from build123d import *

# Parameters (mm, degrees)
F0_W     = 119
F0_H     = 150.5
F1_DEPTH = 22
F2_W     = 109
F2_H     = 140.5
F3_DEPTH = 15
F5_DEPTH = 25
F7_DEPTH = 4


with BuildPart() as f1:
    # F0 (on Front) → F1 (new body)
    with BuildSketch(Plane.XZ):
        Rectangle(F0_W, F0_H)
    extrude(amount=F1_DEPTH)

    # F2 (on face) → F3 (cut)
    with BuildSketch(Plane.XZ.offset(22)):
        Rectangle(F2_W, F2_H)
    extrude(amount=-F3_DEPTH, mode=Mode.SUBTRACT)

    # F4 (on face) → F5 (cut)
    with BuildSketch(Plane.YZ.offset(59.5)):
        Polygon((-22, 65.25), (-22, 0), (-22, -65.25), (-12, -65.25), (-12, 0), (-12, 65.25), align=None)
    extrude(amount=-F5_DEPTH, mode=Mode.SUBTRACT)

    # F6 (on face) → F7 (cut)
    with BuildSketch(Plane.XZ.offset(7)):
        with BuildLine():
            Line((-46.5, 60.75), (-46.5, 65.75))
            ThreePointArc((-46.5, 65.75), (-49, 68.25), (-51.5, 65.75))
            Line((-51.5, 65.75), (-51.5, 60.75))
            ThreePointArc((-51.5, 60.75), (-49, 58.25), (-46.5, 60.75))
        make_face()
        with BuildLine():
            Line((51.5, 61.75), (51.5, 66.75))
            ThreePointArc((51.5, 66.75), (49, 69.25), (46.5, 66.75))
            Line((46.5, 66.75), (46.5, 61.75))
            ThreePointArc((46.5, 61.75), (49, 59.25), (51.5, 61.75))
        make_face()
        with BuildLine():
            Line((46.5, -61.55), (46.5, -66.55))
            ThreePointArc((46.5, -66.55), (49, -69.05), (51.5, -66.55))
            Line((51.5, -66.55), (51.5, -61.55))
            ThreePointArc((51.5, -61.55), (49, -59.05), (46.5, -61.55))
        make_face()
        with BuildLine():
            Line((-52.5, -53.15), (-52.5, -58.15))
            ThreePointArc((-52.5, -58.15), (-50, -60.65), (-47.5, -58.15))
            Line((-47.5, -58.15), (-47.5, -53.524891))
            ThreePointArc((-47.5, -53.524891), (-49.797974, -50.642983), (-52.5, -53.15))
        make_face()
    extrude(amount=-F7_DEPTH, mode=Mode.SUBTRACT)


solid = f1.part
Design review of the part built by this model. Coordinates are the model's own, in mm. A direction names the side the tool comes from. Coordinates: 2 decimals unless noted, no trailing zeros. Order: outer loops, then holes, each group sorted by start corner. A loop starts at its lowest first (then second) coordinate and runs counter-clockwise, first axis right, second up. Notation, with made-up numbers: (86, 55.5) -> (120, 55.5) arc R10 cw to (120, 69.5) -> close; hole circle Ø4 at (16, 76.25). An arc over 180 degrees is marked (long way). One line per item, written item: value.
1) Draft analysis for pull direction X (two halves, no side actions). For faces 4 (the face through (51.5, -5, -64)), 5 (the face through (-59.5, -11, -1)), 6 (the face through (-1, -11, 75.25)), state which applies: +X half, -X half, draft (parallel to the pull), parting line (faces both ways), or undercut.
Output values:
face 4: undercut
face 5: -X half
face 6: draft
2) We need section A-A, the plane y = -9.75. Give the boundary of the cut face in (x, z), then the cut area to 4 significant figures.
Output values:
outline: (-59.5, -75.25) -> (59.5, -75.25) -> (59.5, 75.25) -> (-59.5, 75.25) -> close; hole (-54.5, -70.25) -> (54.5, -70.25) -> (54.5, 70.25) -> (-54.5, 70.25) -> close
area: 2,595 mm2
3) We need section C-C, the plane x = 49. Give the boundary of the cut face in (y, z), then the cut area to 3 significant figures.
Output values:
outline: (-22, -75.25) -> (0, -75.25) -> (0, 75.25) -> (-22, 75.25) -> (-22, 70.25) -> (-7, 70.25) -> (-7, 69.25) -> (-3, 69.25) -> (-3, 59.25) -> (-7, 59.25) -> (-7, -59.05) -> (-3, -59.05) -> (-3, -69.05) -> (-7, -69.05) -> (-7, -70.25) -> (-22, -70.25) -> close
area: 1,120 mm2
4) To check wall thickness, follow probe 1 along Z at (x, y) = (-12, -10.5); probe 2 along X at (y, z) = (-10, -50); probe 3 along Y at (x, z) = (-27, 18). State the ranges of each line that lie inside material, in increasing order. Write a range as [from, to].
Output values:
probe 1: z = [-75.25, -70.25], [70.25, 75.25]
probe 2: x = [-59.5, -54.5], [54.5, 59.5]
probe 3: y = [-7, 0]
5) Machinability: for faces 1 (the face through (-58, -22, 0)), 2 (the face through (-46.5, -5, 63)), 3 (the face through (57, -12, -1)), which of the approach directions +Z, -Z, +X, -X, +Y, -Y give a long, thin tool a straight path to every point of the face, cutting with its end or side? Answer none if there is none.
Output values:
face 1: +Z, -Z, +X, -X, -Y
face 2: -Y
face 3: +X, -Y
6) We need section D-D, the plane x = 14. Give the boundary of the cut face in (y, z).
Output values:
outline: (-22, -75.25) -> (0, -75.25) -> (0, 75.25) -> (-22, 75.25) -> (-22, 70.25) -> (-7, 70.25) -> (-7, -70.25) -> (-22, -70.25) -> close
7) We need section B-B, the plane z = -15.5. Give the boundary of the cut face in (x, y), then the cut area to 3 significant figures.
Output values:
outline: (-59.5, -22) -> (-54.5, -22) -> (-54.5, -7) -> (54.5, -7) -> (54.5, -12) -> (59.5, -12) -> (59.5, 0) -> (-59.5, 0) -> close
area: 933 mm2
8) Clearance check with flat-ended pins moving along their axes: P1, Ø5.5, axis at x = -49.5, z = 62.5, coming from the -Y side; P2, Ø2.5, axis at x = 49.5, z = -66, coming from the -Y side; P3, Ø4.5, axis at y = -17.5, z = -7.5, coming from the +X side. State where each tip first meets the part, or that it passes through.
Output values:
P1: stops at y = -7
P2: stops at y = -3
P3: stops at x = -54.5
